The drawing under review shows one solid part. Ordinate dimensions are in mm from its lowest x, y, z. Coordinates: 2 decimals unless noted, no trailing zeros. Loops run counter-clockwise (first coordinate to the right, second up) from the corner with the lowest first, then second, coordinate; pieces in that order, holes last. Notation, with made-up numbers: (83.25, 87) -> (103.25, 87) arc R20 cw to (103.25, 98) -> close; hole circle Ø7 at (81, 81.5). An arc over 180 degrees is marked (long way). Use a Markdown table: item, result.
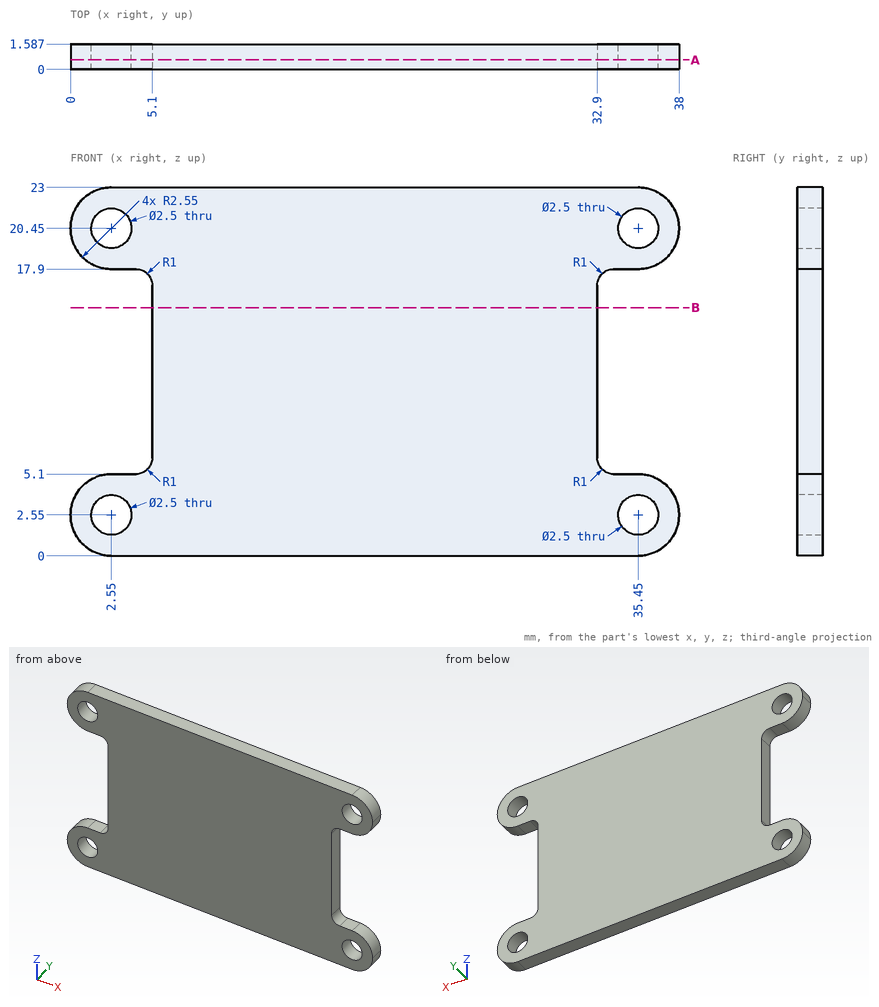
(1) Take a section at A-A on y = 0.6. Write out the cut boundary in (x, z).
Found:
| item | result |
|---|---|
| outline | (2.55, 0) -> (35.45, 0) arc R2.55 ccw to (35.45, 5.1) -> (33.9, 5.1) arc R1 cw to (32.9, 6.1) -> (32.9, 16.9) arc R1 cw to (33.9, 17.9) -> (35.45, 17.9) arc R2.55 ccw to (35.45, 23) -> (2.55, 23) arc R2.55 ccw to (2.55, 17.9) -> (4.1, 17.9) arc R1 cw to (5.1, 16.9) -> (5.1, 6.1) arc R1 cw to (4.1, 5.1) -> (2.55, 5.1) arc R2.55 ccw to start; hole circle Ø2.5 at (2.55, 2.55); hole circle Ø2.5 at (2.55, 20.45); hole circle Ø2.5 at (35.45, 2.55); hole circle Ø2.5 at (35.45, 20.45) |
(2) For line 1 along X through (y, z) = (1.1, 20.45); line 2 along Z through (x, y) = (3.5, 0.9) (1 decimal); line 3 along X through (y, z) = (0.3, 3.25) (1 decimal), list the stretches that pass through material, from the lowest coordinate up.
Found:
| item | result |
|---|---|
| line 1 | x = 0 to 1.3, 3.8 to 34.2, 36.7 to 38 |
| line 2 | z = 0 to 1.7, 3.4 to 5.1, 17.9 to 19.6, 21.3 to 23 |
| line 3 | x = 0.1 to 1.5, 3.6 to 34.4, 36.5 to 37.9 |
(3) For pin 1 Ø0.5 at (y, z) = (0.5, 12) entering from -X, flat-tipped, find the tip position at first contact; note if it passes through.
Found:
| item | result |
|---|---|
| pin 1 | stops at x = 5.1 |
(4) Take a section at B-B on z = 15.5. Write out the cut boundary in (x, y).
Found:
| item | result |
|---|---|
| outline | (5.1, 0) -> (32.9, 0) -> (32.9, 1.59) -> (5.1, 1.59) -> close |
